Work out the finished part from the listing and answer in its coordinate system (mm). A direction names the side the tool comes from. Round coordinates to 2 decimals unless told otherwise and drop trailing zeros. Write each loop counter-clockwise with the first axis right and the second up, starting at its lowest first coordinate (ties: lowest second). Pieces come first, ordered by that corner, then holes.
1. A flat-ended cylindrical pin translates along its axis: pin 1 Ø10 at (y, z) = (-13, 39.5) entering from -X. Find the tip coordinate at first contact, or state that the pin passes through.
2. Determine the mould class of faces 1 (the face through (85.885, -11, 35)), 2 (the face through (48.93, -44.39, 32.69)), 3 (the face through (9, -42.363, 35)) for opening direction X: pulls with the +X half, pulls with the -X half, needs draft (parallel to the pull), parting line crosses it, or undercut.
3. Find section B-B (x = 39.5). Write down the section's boundary in (y, z), and give its area (3 significant figures).
4. Find section D-D (z = 26). Write down the section's boundary in (x, y), and give its area (3 significant figures).
5. Find section C-C (y = -18.5). Write down the section's boundary in (x, z).
6. A tool of negligible diameter and unlimited length cuts with its end or side. For faces 4 (the face through (9, 19.637, 35)), 5 (the face through (-58.007, -44.391, 33.656)), 6 (the face through (-65.115, -43, 30)), from which of +Z, -Z, +X, -X, +Y, -Y can it reach the whole face along a straight path? Write none if from no direction.
7. Find section A-A (z = 35). Write down the section's boundary in (x, y).
8. Straight lines are drawn through the part: probe 1 along X at (y, z) = (-44.2, 35); probe 2 along Z at (x, y) = (-5.5, -7); probe 3 along Y at (x, z) = (-54, 44.5). For each, find the intervals that lie inside material, in ascending order.
```python
from build123d import *

# Parameters (mm, degrees)
ESQUISSE1_W             = 155
ESQUISSE1_H             = 70
BOSS_EXTRU_1_DEPTH      = 70
ESQUISSE2_W             = 62
ESQUISSE2_H             = 62
ENL_V_MAT_EXTRU_1_DEPTH = 151
ESQUISSE3_R             = 2.5
ENL_V_MAT_EXTRU_2_DEPTH = 5


with BuildPart() as part:
    # Esquisse1 → Boss.-Extru.1 (new body)
    with BuildSketch(Plane.XY):
        with Locations((12.385350745, -11.363216266)):
            Rectangle(ESQUISSE1_W, ESQUISSE1_H)
    extrude(amount=BOSS_EXTRU_1_DEPTH)

    # Esquisse2 → Enlèv. mat.-Extru.1 (cut)
    with BuildSketch(Plane.ZY.offset(65.114649255)):
        with Locations((35, -11.363216266)):
            Rectangle(ESQUISSE2_W, ESQUISSE2_H)
    extrude(amount=-ENL_V_MAT_EXTRU_1_DEPTH, mode=Mode.SUBTRACT)

    # Esquisse3 → Enlèv. mat.-Extru.2 (cut)
    with BuildSketch(Plane.XZ.offset(46.363216266)):
        with Locations(Location((-60.114649255, 35, 0), (0, 0, 270))):
            Circle(ESQUISSE3_R)
        with Locations(Location((49.885350745, 35, 0), (0, 0, 270))):
            Circle(ESQUISSE3_R)
    extrude(amount=-ENL_V_MAT_EXTRU_2_DEPTH, mode=Mode.SUBTRACT)


solid = part.part
```
Worked answers:
1. pin 1: stops at x = 85.89
2. face 1: pulls with the -X half
2. face 2: undercut
2. face 3: needs draft
3. outline: (-46.36, 0) - (23.64, 0) - (23.64, 70) - (-46.36, 70) - close; hole (-42.36, 4) - (19.64, 4) - (19.64, 66) - (-42.36, 66) - close
3. area: 1,060 mm2
4. outline: (-65.11, -46.36) - (89.89, -46.36) - (89.89, 23.64) - (-65.11, 23.64) - (-65.11, 19.64) - (85.89, 19.64) - (85.89, -42.36) - (-65.11, -42.36) - close
4. area: 1,490 mm2
5. outline: (-65.11, 0) - (89.89, 0) - (89.89, 70) - (-65.11, 70) - (-65.11, 66) - (85.89, 66) - (85.89, 4) - (-65.11, 4) - close
6. face 4: -X
6. face 5: -Y
6. face 6: +Z, -Z, -X, +Y, -Y
7. outline: (-65.11, -46.36) - (-62.61, -46.36) - (-62.61, -42.36) - (-65.11, -42.36) - close; (-65.11, 19.64) - (85.89, 19.64) - (85.89, -42.36) - (52.39, -42.36) - (52.39, -46.36) - (89.89, -46.36) - (89.89, 23.64) - (-65.11, 23.64) - close; (-57.61, -46.36) - (47.39, -46.36) - (47.39, -42.36) - (-57.61, -42.36) - close
8. probe 1: x = -65.11 to -62.61, -57.61 to 47.39, 52.39 to 89.89
8. probe 2: z = 0 to 4, 66 to 70
8. probe 3: y = -46.36 to -42.36, 19.64 to 23.64
